Verification items for the finished model (mm, model axes). A direction names the side the tool comes from. Coordinates: 2 decimals unless noted, no trailing zeros. Order: outer loops, then holes, each group sorted by start corner. A loop starts at its lowest first (then second) coordinate and runs counter-clockwise, first axis right, second up. Notation, with made-up numbers: M 85.25,61.5 L 141.25,61.5 A23 ccw 141.25,99.5 Z; hole C 43,40 d1. An arc over 180 degrees is marked long. Return JSON: item names as keys, results as strings. Group by question number.
1. Section check B-B, the plane x = -7.5. Record the cut outline in (y, z).
2. Set-up check for faces 4 (the cylindrical face through (-13.92, 17.31, -8.68)), 5 (the flat face through (-17.975, 33, 7)): record each of +Z, -Z, +X, -X, +Y, -Y from which the full face is reachable in a straight line by a thin tool's end or side.
3. Material ranges on line 1 along Z through (x, y) = (15, 24); line 2 along X through (y, z) = (34, -7.5); line 3 along Y through (x, z) = (17.5, -8.25), recorded low to high.
4. Section check D-D, the plane z = 1.25. Record the cut outline in (x, y).
5. Mould release check, pull along Z, two halves, no side actions. Record for faces 1 (the flat face through (22.5, 17, 0)), 2 (the cylindrical face through (16.586, 34.366, -7.708)), 3 (the flat face through (16, 3.75, 9)): +Z half, -Z half, draft (parallel to the pull), parting line (faces both ways), or undercut.
6. Gauge pin test, flat ends, axial feed: pin 1 (13.5 mm diameter, centred on x = -7.5, y = 17.5, fed in from -Z); pin 2 (3 mm diameter, centred on x = 15, z = -7.5, fed in from +Y). Record the tip position at first contact, or that the pin passes through.
7. Section check A-A, the plane y = 17.5. Record the cut outline in (x, z).
8. Section check C-C, the plane z = -7.5. Give the number of separate pieces and of enclosed holes in the cut face, plus the area to 3 significant figures.
```python
from build123d import *

# Parameters (mm, degrees)
SKETCH1_W           = 15
SKETCH1_H           = 30
SKETCH1_R           = 1.6
BOSS_EXTRUDE1_DEPTH = 5
CUT_EXTRUDE1_START  = 1.25
SKETCH1_3_R         = 1.6
CUT_EXTRUDE1_DEPTH  = 2.5
BOSS_EXTRUDE2_START = 5
SKETCH1_4_W         = 15
SKETCH1_4_H         = 30
SKETCH1_4_R         = 1.6
BOSS_EXTRUDE2_DEPTH = 30
SKETCH5_R           = 4.15
CUT_EXTRUDE2_DEPTH  = 52.295711322
CUT_EXTRUDE3_START  = -1.25
CUT_EXTRUDE3_DEPTH  = 2.5


with BuildPart() as part:
    # Sketch1 → Boss-Extrude1 (new body)
    with BuildSketch(Plane(origin=(0, 0, 0), x_dir=(1, 0, 0), z_dir=(0, 1, 0))):
        with Locations((-15, 0)):
            Rectangle(SKETCH1_W, SKETCH1_H)
        Polygon((-12.025, -5.782382949), (-15, -4.064765898), (-17.975, -5.782382949), (-17.975, -9.217617051), (-15, -10.935234102), (-12.025, -9.217617051), align=None, mode=Mode.SUBTRACT)
        Polygon((-12.025, 9.217617051), (-15, 10.935234102), (-17.975, 9.217617051), (-17.975, 5.782382949), (-15, 4.064765898), (-12.025, 5.782382949), align=None, mode=Mode.SUBTRACT)
        Rectangle(SKETCH1_W, SKETCH1_H)
        with Locations((15, 0)):
            Rectangle(SKETCH1_W, SKETCH1_H)
        Polygon((17.975, -5.782382949), (15, -4.064765898), (12.025, -5.782382949), (12.025, -9.217617051), (15, -10.935234102), (17.975, -9.217617051), align=None, mode=Mode.SUBTRACT)
        Polygon((17.975, 9.217617051), (15, 10.935234102), (12.025, 9.217617051), (12.025, 5.782382949), (15, 4.064765898), (17.975, 5.782382949), align=None, mode=Mode.SUBTRACT)
        Polygon((-12.025, -9.217617051), (-12.025, -5.782382949), (-15, -4.064765898), (-17.975, -5.782382949), (-17.975, -9.217617051), (-15, -10.935234102), align=None)
        with Locations(Location((-15, -7.5, 0), (0, 0, 270))):
            Circle(SKETCH1_R, mode=Mode.SUBTRACT)
        Polygon((-12.025, 5.782382949), (-12.025, 9.217617051), (-15, 10.935234102), (-17.975, 9.217617051), (-17.975, 5.782382949), (-15, 4.064765898), align=None)
        with Locations(Location((-15, 7.5, 0), (0, 0, 270))):
            Circle(SKETCH1_R, mode=Mode.SUBTRACT)
        Polygon((17.975, 5.782382949), (17.975, 9.217617051), (15, 10.935234102), (12.025, 9.217617051), (12.025, 5.782382949), (15, 4.064765898), align=None)
        with Locations(Location((15, 7.5, 0), (0, 0, 270))):
            Circle(SKETCH1_R, mode=Mode.SUBTRACT)
        Polygon((17.975, -9.217617051), (17.975, -5.782382949), (15, -4.064765898), (12.025, -5.782382949), (12.025, -9.217617051), (15, -10.935234102), align=None)
        with Locations(Location((15, -7.5, 0), (0, 0, 270))):
            Circle(SKETCH1_R, mode=Mode.SUBTRACT)
    extrude(amount=BOSS_EXTRUDE1_DEPTH)

    # Sketch1<3> → Cut-Extrude1 (cut)
    with BuildSketch(Plane(origin=(0, 0, 0), x_dir=(1, 0, 0), z_dir=(0, 1, 0)).offset(CUT_EXTRUDE1_START)):
        Polygon((-12.025, 5.782382949), (-12.025, 9.217617051), (-15, 10.935234102), (-17.975, 9.217617051), (-17.975, 5.782382949), (-15, 4.064765898), align=None)
        with Locations(Location((-15, 7.5, 0), (0, 0, 270))):
            Circle(SKETCH1_3_R, mode=Mode.SUBTRACT)
        Polygon((-12.025, -9.217617051), (-12.025, -5.782382949), (-15, -4.064765898), (-17.975, -5.782382949), (-17.975, -9.217617051), (-15, -10.935234102), align=None)
        with Locations(Location((-15, -7.5, 0), (0, 0, 270))):
            Circle(SKETCH1_3_R, mode=Mode.SUBTRACT)
        Polygon((17.975, -9.217617051), (17.975, -5.782382949), (15, -4.064765898), (12.025, -5.782382949), (12.025, -9.217617051), (15, -10.935234102), align=None)
        with Locations(Location((15, -7.5, 0), (0, 0, 270))):
            Circle(SKETCH1_3_R, mode=Mode.SUBTRACT)
        Polygon((17.975, 5.782382949), (17.975, 9.217617051), (15, 10.935234102), (12.025, 9.217617051), (12.025, 5.782382949), (15, 4.064765898), align=None)
        with Locations(Location((15, 7.5, 0), (0, 0, 270))):
            Circle(SKETCH1_3_R, mode=Mode.SUBTRACT)
    extrude(amount=CUT_EXTRUDE1_DEPTH, mode=Mode.SUBTRACT)

    # Sketch1<4> → Boss-Extrude2 (add)
    with BuildSketch(Plane(origin=(0, 0, 0), x_dir=(1, 0, 0), z_dir=(0, 1, 0)).offset(BOSS_EXTRUDE2_START)):
        Rectangle(SKETCH1_4_W, SKETCH1_4_H)
        with Locations((-15, 0)):
            Rectangle(SKETCH1_4_W, SKETCH1_4_H)
        Polygon((-12.025, -5.782382949), (-15, -4.064765898), (-17.975, -5.782382949), (-17.975, -9.217617051), (-15, -10.935234102), (-12.025, -9.217617051), align=None, mode=Mode.SUBTRACT)
        Polygon((-12.025, 9.217617051), (-15, 10.935234102), (-17.975, 9.217617051), (-17.975, 5.782382949), (-15, 4.064765898), (-12.025, 5.782382949), align=None, mode=Mode.SUBTRACT)
        Polygon((-12.025, -9.217617051), (-12.025, -5.782382949), (-15, -4.064765898), (-17.975, -5.782382949), (-17.975, -9.217617051), (-15, -10.935234102), align=None)
        with Locations(Location((-15, -7.5, 0), (0, 0, 270))):
            Circle(SKETCH1_4_R, mode=Mode.SUBTRACT)
        Polygon((-12.025, 5.782382949), (-12.025, 9.217617051), (-15, 10.935234102), (-17.975, 9.217617051), (-17.975, 5.782382949), (-15, 4.064765898), align=None)
        with Locations(Location((-15, 7.5, 0), (0, 0, 270))):
            Circle(SKETCH1_4_R, mode=Mode.SUBTRACT)
        with Locations((15, 0)):
            Rectangle(SKETCH1_4_W, SKETCH1_4_H)
        Polygon((17.975, -5.782382949), (15, -4.064765898), (12.025, -5.782382949), (12.025, -9.217617051), (15, -10.935234102), (17.975, -9.217617051), align=None, mode=Mode.SUBTRACT)
        Polygon((17.975, 9.217617051), (15, 10.935234102), (12.025, 9.217617051), (12.025, 5.782382949), (15, 4.064765898), (17.975, 5.782382949), align=None, mode=Mode.SUBTRACT)
        Polygon((17.975, -9.217617051), (17.975, -5.782382949), (15, -4.064765898), (12.025, -5.782382949), (12.025, -9.217617051), (15, -10.935234102), align=None)
        with Locations(Location((15, -7.5, 0), (0, 0, 270))):
            Circle(SKETCH1_4_R, mode=Mode.SUBTRACT)
        Polygon((17.975, 5.782382949), (17.975, 9.217617051), (15, 10.935234102), (12.025, 9.217617051), (12.025, 5.782382949), (15, 4.064765898), align=None)
        with Locations(Location((15, 7.5, 0), (0, 0, 270))):
            Circle(SKETCH1_4_R, mode=Mode.SUBTRACT)
    extrude(amount=BOSS_EXTRUDE2_DEPTH)

    # Sketch5 → Cut-Extrude2 (cut, through all)
    with BuildSketch(Plane.XY.offset(15)):
        with Locations((-7.5, 17.5)):
            Circle(SKETCH5_R)
        with Locations((7.5, 17.5)):
            Circle(SKETCH5_R)
    extrude(amount=-CUT_EXTRUDE2_DEPTH, mode=Mode.SUBTRACT)

    # Sketch6 → Cut-Extrude3 (cut)
    with BuildSketch(Plane(origin=(0, 35, 0), x_dir=(1, 0, 0), z_dir=(0, 1, 0)).offset(CUT_EXTRUDE3_START)):
        Polygon((-15, 10.935234102), (-17.975, 9.217617051), (-17.975, 5.782382949), (-15, 4.064765898), (-12.025, 5.782382949), (-12.025, 9.217617051), align=None)
        Polygon((15, 10.935234102), (12.025, 9.217617051), (12.025, 5.782382949), (15, 4.064765898), (17.975, 5.782382949), (17.975, 9.217617051), align=None)
        Polygon((15, -4.064765898), (12.025, -5.782382949), (12.025, -9.217617051), (15, -10.935234102), (17.975, -9.217617051), (17.975, -5.782382949), align=None)
        Polygon((-15, -4.064765898), (-17.975, -5.782382949), (-17.975, -9.217617051), (-15, -10.935234102), (-12.025, -9.217617051), (-12.025, -5.782382949), align=None)
    extrude(amount=-CUT_EXTRUDE3_DEPTH, mode=Mode.SUBTRACT)


solid = part.part
```
Answers follow:
{
 "1": {"outline": "M 0,-15 L 13.35,-15 L 13.35,15 L 0,15 Z; M 21.65,-15 L 35,-15 L 35,15 L 21.65,15 Z"},
 "2": {"face 4": "+Y, -Y", "face 5": "none"},
 "3": {"line 1": "-15 to -9.1, -5.9 to 5.9, 9.1 to 15", "line 2": "-22.5 to -16.6, -13.4 to 13.4, 16.6 to 22.5", "line 3": "0 to 1.25, 3.75 to 31.25, 33.75 to 35"},
 "4": {"outline": "M -22.5,0 L 22.5,0 L 22.5,35 L -22.5,35 Z; hole C -7.5,17.5 d8.3; hole C 7.5,17.5 d8.3"},
 "5": {"face 1": "draft", "face 2": "undercut", "face 3": "undercut"},
 "6": {"pin 1": "z = -15", "pin 2": "through"},
 "7": {"outline": "M -22.5,-15 L -11.65,-15 L -11.65,15 L -22.5,15 Z; M -3.35,-15 L 3.35,-15 L 3.35,15 L -3.35,15 Z; M 11.65,-15 L 22.5,-15 L 22.5,15 L 11.65,15 Z; hole C -15,-7.5 d3.2; hole C -15,7.5 d3.2; hole C 15,-7.5 d3.2; hole C 15,7.5 d3.2"},
 "8": {"separate pieces": "3", "enclosed holes": "2", "area": "1,220 mm^2"}
}
